Could you check a few things on this model? Use its own coordinates, in mm. Face numbers are marked on the shaded views. Round coordinates to 2 decimals unless told otherwise and drop trailing zeros. Loops run counter-clockwise (first coordinate to the right, second up) from the corner with the lowest first, then second, coordinate; pieces in that order, holes last. Notation, with made-up numbers: (-23, -3.5) - (17, -3.5) arc R20 ccw to (17, 11.5) - close; hole circle Ø11 at (41, 61). An arc over 180 degrees is marked (long way). Put each result on its own line as item: value. Start each with the question number.
from build123d import *

# Parameters (mm, degrees)
F2_R = 3.81
F3_R = 1.524
F5_R = 4.7625


with BuildPart() as f1:
    # F0 (on Front) → F1 (revolve)
    with BuildSketch(Plane.XZ):
        Polygon((0, 76.2), (0, 0), (20.32, 0), (17.78, 9.525), (14.224, 9.525), (14.224, 25.4), (16.51, 25.4), (16.51, 76.2), align=None)
    revolve(axis=Axis((0, 0, 38.1), (0, 0, 1)))

    # F2
    f2_edges = [f1.edges().sort_by_distance(p)[0] for p in [
        (-16.51, 0, 76.2),
    ]]
    fillet(f2_edges, radius=F2_R)

    # F3
    f3_edges = [f1.edges().sort_by_distance(p)[0] for p in [
        (-17.78, 0, 9.525),
    ]]
    fillet(f3_edges, radius=F3_R)

    # F6: sweep along a path in F4
    with BuildLine(Plane.YZ) as f6_path:
        Line((0, 60.96), (-44.7385872582, 73.66))
        ThreePointArc((-44.7385872582, 73.66), (-63.5228620001, 73.5779674415), (-79.375, 63.5))
    # F5 (on Front) → F6 (sweep)
    with BuildSketch(Plane.XZ):
        with Locations((0, 60.96)):
            Circle(F5_R)
    sweep(path=f6_path.line)


solid = f1.part
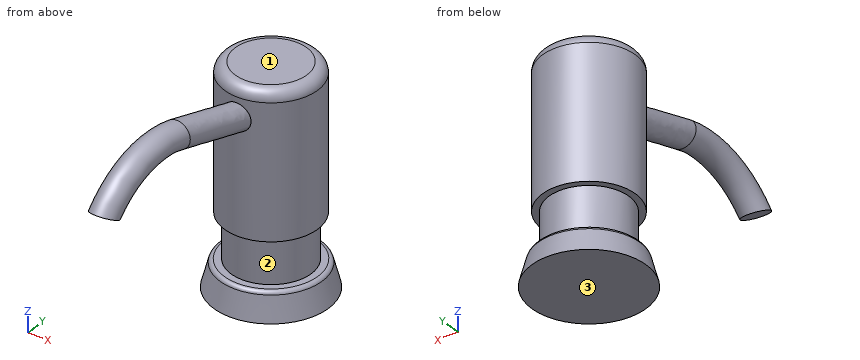
Item 1: Suppose I cut it at C-C, the plane z = 19.5. List the corners of the cut face in (x, y) for me, then the cut area to 3 significant figures.
Item 2: I need wall thicknesses on line 1 (Z direction, x = -11, y = -3); line 2 (Z direction, x = 12.5, y = 11); line 3 (Y direction, x = -10.5, z = 35.5). Which ranges of each line are inside material? Lowest first, please. Write a range as from..to.
Item 3: Will these pins go through, and if not, where does the flat tip stop? P1, Ø3, axis at x = 1, y = -34, coming from the -Z side; P2, Ø10, axis at x = -4.5, y = 5.5, coming from the -Z side; P3, Ø5, axis at x = 6, y = -63, coming from the -Z side; P4, Ø16.5, axis at x = 0, y = -3, coming from the +Z side.
Item 4: Thinking about a two-plate mould opening in Z: for the marked faces 1, 2 and 3, which applies, released by +Z, released by -Z, zero draft, split by the parting line, or undercut?
Item 5: Suppose I cut it at B-B, the plane z = 36. List the corners of the cut face in (x, y) for me, then the cut area to 3 significant figures.
Item 6: Suppose I cut it at A-A, the plane y = 0. List the corners of the cut face in (x, z) for me (3 decimals), then the cut area to 3 significant figures.
Numbers:
1. outline: circle Ø28.45 at (0, 0)
1. area: 636 mm^2
2. line 1: 0..76.2
2. line 2: 0..9.52
2. line 3: -12.74..12.74
3. P1: z = 65.47
3. P2: z = 0
3. P3: z = 70.39
3. P4: z = 76.2
4. face 1: released by +Z
4. face 2: undercut
4. face 3: released by -Z
5. outline: circle Ø33.02 at (0, 0)
5. area: 856 mm^2
6. outline: (-20.32, 0) - (20.32, 0) - (18.082, 8.394) arc R1.524 ccw to (16.609, 9.525) - (14.224, 9.525) - (14.224, 25.4) - (16.51, 25.4) - (16.51, 72.39) arc R3.81 ccw to (12.7, 76.2) - (-12.7, 76.2) arc R3.81 ccw to (-16.51, 72.39) - (-16.51, 25.4) - (-14.224, 25.4) - (-14.224, 9.525) - (-16.609, 9.525) arc R1.524 ccw to (-18.082, 8.394) - close
6. area: 2,490 mm^2
